Autodesk Inventor part; units mm, degrees
ref_plane "YZ Plane" through (0, 0, 0) normal (1, 0, 0) x (0, 1, 0)
ref_plane "XZ Plane" through (0, 0, 0) normal (0, 1, 0) x (-1, 0, 0)
ref_plane "XY Plane" through (0, 0, 0) normal (0, 0, 1) x (1, 0, 0)
sketch "Sketch1" plane through (0, 0, 0) normal (0, 1, 0) x (-1, 0, 0)
  line L0 (146.1818, 19) -> (146.1818, 22)
  line L1 (114.3636, 22) -> (114.3636, 19)
  line L2 (82.5455, 19) -> (82.5455, 22)
  line L3 (50.7273, 22) -> (50.7273, 19)
  line L4 (18.9091, 19) -> (18.9091, 22)
  line L5 (-12.9091, 22) -> (-12.9091, 19)
  line L6 (-44.7273, 19) -> (-44.7273, 22)
  line L7 (-76.5455, 22) -> (-76.5455, 19)
  line L8 (-108.3636, 19) -> (-108.3636, 22)
  line L9 (-140.1818, 22) -> (-140.1818, 19)
  line L10 (-172, 15) -> (-169, 15)
  line L11 (-169, 3) -> (-172, 3)
  line L12 (-169, -9) -> (-172, -9)
  line L13 (-172, -21) -> (-169, -21)
  line L14 (-140.1818, -25) -> (-140.1818, -28)
  line L15 (-108.3636, -28) -> (-108.3636, -25)
  line L16 (-76.5455, -25) -> (-76.5455, -28)
  line L17 (-44.7273, -28) -> (-44.7273, -25)
  line L18 (-12.9091, -28) -> (-12.9091, -25)
  line L19 (18.9091, -25) -> (18.9091, -28)
  line L20 (146.1818, -28) -> (146.1818, -25)
  line L21 (114.3636, -25) -> (114.3636, -28)
  line L22 (82.5455, -28) -> (82.5455, -25)
  line L23 (50.7273, -25) -> (50.7273, -28)
  line L24 (178, -21) -> (175, -21)
  line L25 (175, 15) -> (178, 15)
  line L26 (178, 3) -> (175, 3)
  line L27 (114.3636, -28) -> (146.1818, -28)
  line L28 (50.7273, -28) -> (82.5455, -28)
  line L29 (-12.9091, -28) -> (18.9091, -28)
  line L30 (178, -21) -> (178, -17)
  line L31 (178, 3) -> (178, 7)
  line L32 (178, 11) -> (178, 15)
  line L33 (146.1818, 22) -> (114.3636, 22)
  line L34 (82.5455, 22) -> (50.7273, 22)
  line L35 (18.9091, 22) -> (-12.9091, 22)
  line L36 (-44.7273, 22) -> (-76.5455, 22)
  line L37 (-108.3636, 22) -> (-140.1818, 22)
  line L38 (-169, 15) -> (-169, 11)
  line L39 (-169, 7) -> (-169, 3)
  line L40 (-172, 3) -> (-172, -1)
  line L41 (-172, 19) -> (-172, 15)
  line L42 (-140.1818, -28) -> (-108.3636, -28)
  line L43 (-76.5455, -28) -> (-44.7273, -28)
  line L44 (-169, -9) -> (-169, -13)
  line L45 (-169, -17) -> (-169, -21)
  line L46 (-172, -5) -> (-172, -9)
  line L47 (-172, -21) -> (-172, -25)
  line L48 (-172, -25) -> (-140.1818, -25)
  line L49 (-108.3636, -25) -> (-76.5455, -25)
  line L50 (-44.7273, -25) -> (-12.9091, -25)
  line L51 (18.9091, -25) -> (50.7273, -25)
  line L52 (82.5455, -25) -> (114.3636, -25)
  line L53 (146.1818, -25) -> (175, -25)
  line L54 (175, -25) -> (175, -21)
  line L55 (175, -1) -> (175, 3)
  line L56 (175, 15) -> (175, 19)
  line L57 (175, 19) -> (146.1818, 19)
  line L58 (114.3636, 19) -> (82.5455, 19)
  line L59 (50.7273, 19) -> (18.9091, 19)
  line L60 (-12.9091, 19) -> (-44.7273, 19)
  line L61 (-76.5455, 19) -> (-108.3636, 19)
  line L62 (-140.1818, 19) -> (-172, 19)
  line L63 (178, -13) -> (178, -9)
  line L64 (178, -9) -> (175, -9)
  line L65 (175, -9) -> (175, -5)
  line L66 (-169, -17) -> (-169, -13)
  line L67 (-172, -5) -> (-172, -1)
  line L68 (-169, 7) -> (-169, 11)
  line L69 (178, -17) -> (178, -13)
  line L70 (175, -5) -> (175, -1)
  line L71 (178, 7) -> (178, 11)
  point P0 (0, 0)
  point P1 (-219, 16.6364)
  point P2 (-222, -22.6364)
  point P3 (228, -22.6364)
  dimension "d1" = 347
  dimension "d3" = 44
  dimension "d5" = 25
  dimension "d6" = 175
  dimension "d9" = 3
  dimension "d15" = 3
  dimension "d16" = 3
  dimension "d17" = 3
  dimension "d18" = 12
  dimension "d19" = 12
  dimension "d20" = 12
  dimension "d21" = 4
  dimension "d23" = 31.8182
extrude "Extrusion1" add sketch "Sketch1" along normal blind 3
equation "\"d1\" = wt - tt"
equation "\"d3\" = -2 * tt + ht"
equation "\"d9\" = tt"
equation "\"d15\" = tt"
equation "\"d16\" = tt"
equation "\"d17\" = tt"
equation "\"d18\" = 0.272727 * ht - 0.545455 * tt"
equation "\"d19\" = d18"
equation "\"d20\" = d18"
equation "\"d21\" = -0.181818 * tt + 0.0909091 * ht"
equation "\"d23\" = 0.0909091 * wt"
equation "\"d13\" = tt"
equation "\"wt\" = 350"
equation "\"tt\" = 3"
equation "\"tol\" = 0"
equation "\"tiroir\" = 25.4"
equation "\"nHoles\" = 101.6"
equation "\"shelfH\" = 35"
equation "\"d0\" = 0.5 * wt"
equation "\"d2\" = 0.5 * lt"
equation "\"d4\" = tt"
properties part number "base"
Geometry: final body of the model. Coordinates: model frame, mm. Give positions to 0.01 mm unless a question says otherwise; leave off trailing zeros. Write each loop counter-clockwise with the first axis right and the second up, starting at its lowest first coordinate (ties: lowest second). Pieces come first, ordered by that corner, then holes.
1. Section query A-A, the plane x = 151.5. Return loops of the section in (y, z), then the cut area to 3 significant figures.
2. Line query: probe 1 along Z at (x, y) = (-21, 2.5); probe 2 along X at (y, z) = (1.7, 0.5); probe 3 along X at (y, z) = (0.7, -16). Output: solid intervals per line, ascending.
3. Pin query (flat end, axial travel): P1, Ø1.5, axis at x = -30, y = 1.5, coming from the +Z side; P2, Ø1.5, axis at y = 1, z = 20.5, coming from the -X side; P3, Ø0.9, axis at y = 1.5, z = 20, coming from the +X side. Return the tip coordinate at first contact, or that it passes through.
Computed:
1. outline: (0, -25) - (3, -25) - (3, 19) - (0, 19) - close
1. area: 132 mm2
2. probe 1: z = -25 to 19
2. probe 2: x = -175 to 172
2. probe 3: x = -178 to 169
3. P1: stops at z = 19
3. P2: stops at x = -146.18
3. P3: stops at x = 140.18
